Geometry: see drawing. Coordinates: mm, zero at the bounding-box minimum. Coordinates: 2 decimals unless noted, no trailing zeros. Write each loop counter-clockwise with the first axis right and the second up, starting at its lowest first coordinate (ties: lowest second). Pieces come first, ordered by that corner, then holes.
1) Section query B-B (z = 18). Output: boundary loops of the cut face in (x, y), then the cut area to 3 significant figures.
2) Section query D-D (x = 50.5). Output: boundary loops of the cut face in (y, z), then the cut area to 3 significant figures.
3) Line query: L1, parallel to X at y = 1, z = 18; L2, parallel to Z at x = 29.5, y = 2.05; L3, parallel to Z at x = 40.5, y = 1.75. Output: solid intervals per line, ascending.
4) Section query C-C (y = 0.65). Output: boundary loops of the cut face in (x, z), then the cut area to 3 significant figures.
5) Pin query (flat end, axial travel): pin 1 Ø0.9 at (x, y) = (10, 1) entering from -Z; pin 2 Ø0.8 at (y, z) = (1, 2.5) entering from +X. Return the tip coordinate at first contact, or that it passes through.
6) Section query A-A (x = 29.5). Output: boundary loops of the cut face in (y, z), then the cut area to 3 significant figures.
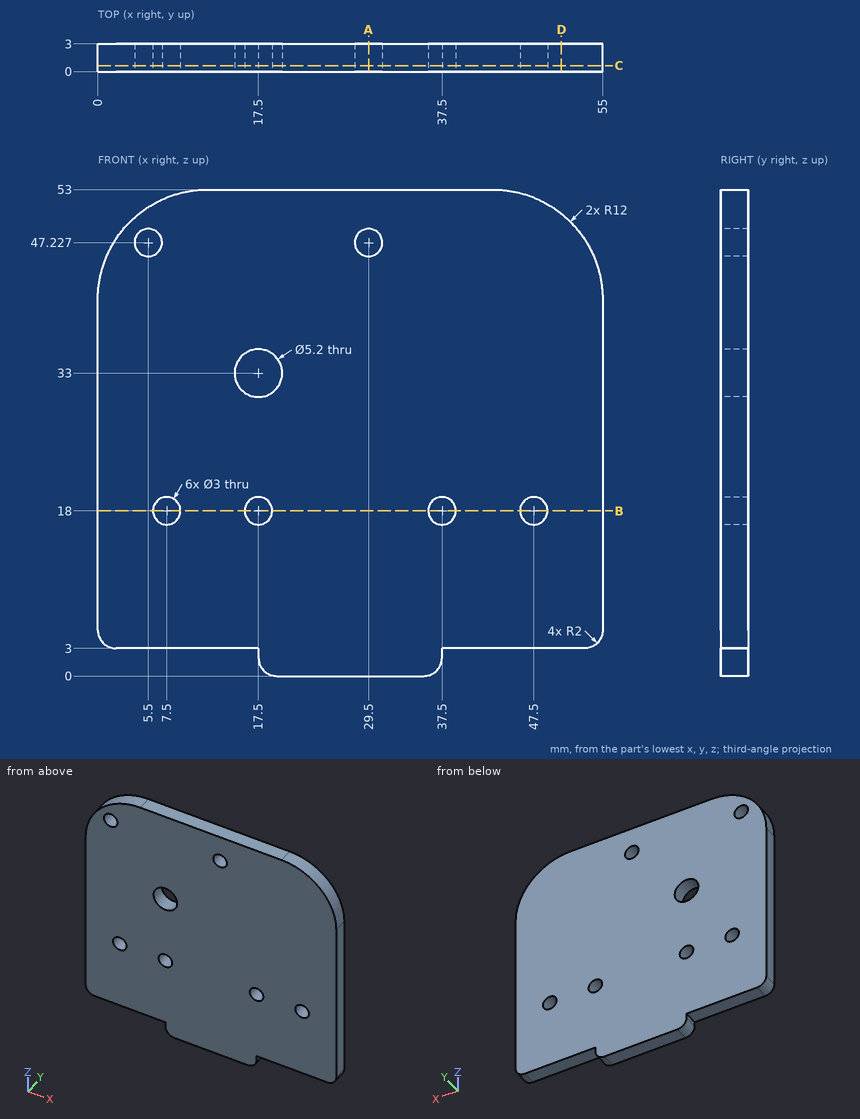
Answer:
1. outline: (0, 0) - (6, 0) - (6, 3) - (0, 3) - close; (9, 0) - (16, 0) - (16, 3) - (9, 3) - close; (19, 0) - (36, 0) - (36, 3) - (19, 3) - close; (39, 0) - (46, 0) - (46, 3) - (39, 3) - close; (49, 0) - (55, 0) - (55, 3) - (49, 3) - close
1. area: 129 mm2
2. outline: (0, 3) - (3, 3) - (3, 50.37) - (0, 50.37) - close
2. area: 142 mm2
3. L1: x = 0 to 6, 9 to 16, 19 to 36, 39 to 46, 49 to 55
3. L2: z = 0 to 45.73, 48.73 to 53
3. L3: z = 3 to 53
4. outline: (0, 5) arc R2 ccw to (2, 3) - (17.5, 3) - (17.5, 2) arc R2 ccw to (19.5, 0) - (35.5, 0) arc R2 ccw to (37.5, 2) - (37.5, 3) - (53, 3) arc R2 ccw to (55, 5) - (55, 41) arc R12 ccw to (43, 53) - (12, 53) arc R12 ccw to (0, 41) - close; hole circle Ø3 at (5.5, 47.23); hole circle Ø3 at (7.5, 18); hole circle Ø5.2 at (17.5, 33); hole circle Ø3 at (17.5, 18); hole circle Ø3 at (29.5, 47.23); hole circle Ø3 at (37.5, 18); hole circle Ø3 at (47.5, 18)
4. area: 2,680 mm2
5. pin 1: stops at z = 3
5. pin 2: stops at x = 37.5
6. outline: (0, 0) - (3, 0) - (3, 45.73) - (0, 45.73) - close; (0, 48.73) - (3, 48.73) - (3, 53) - (0, 53) - close
6. area: 150 mm2
